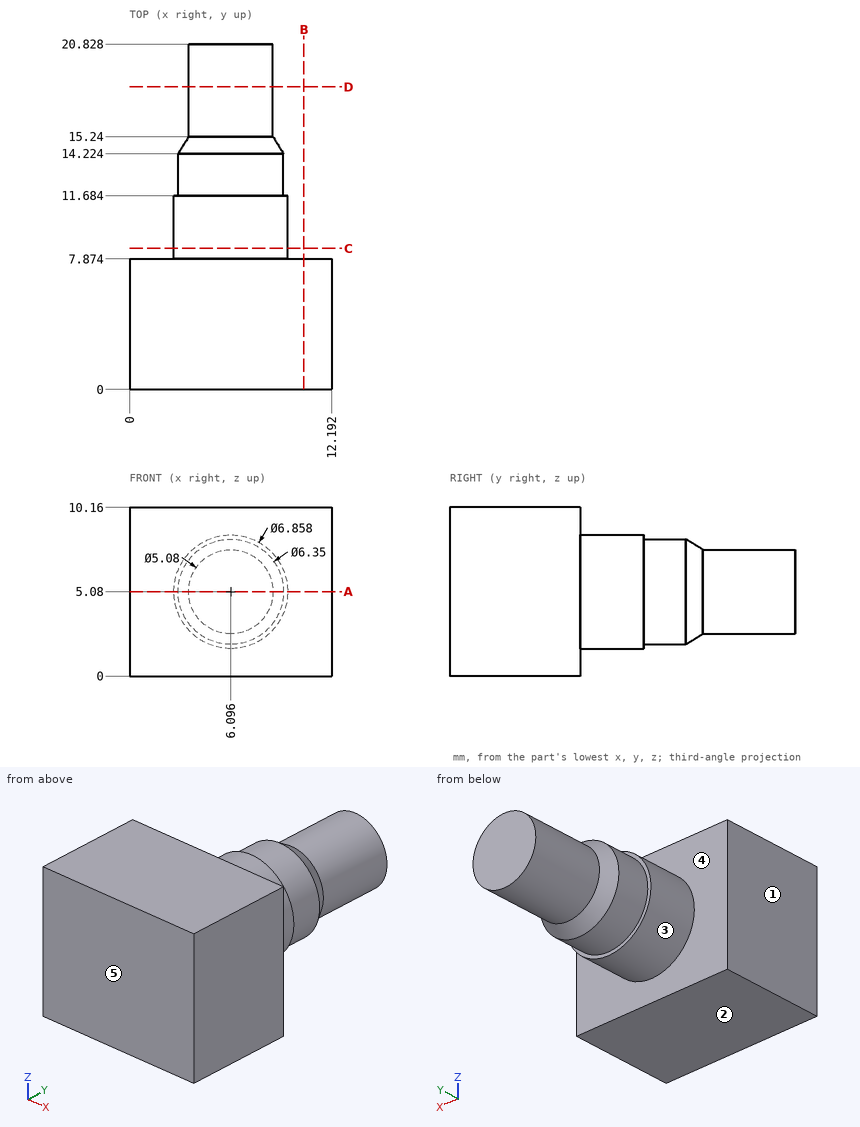
For this review, use the dimensioned drawing (mm, ordinates from the lowest corner) and the shaded views. A direction names the side the tool comes from. Give positions to 0.01 mm unless a question says otherwise; leave off trailing zeros. Order: outer loops, then holes, each group sorted by start corner. A loop starts at its lowest first (then second) coordinate and runs counter-clockwise, first axis right, second up.
1. Mouldability with a two-part tool opening along X and no side actions: class the marked faces 1, 2 and 3 as +X half, -X half, draft (parallel to the pull), parting line (faces both ways), or undercut.
Solution:
face 1: -X half
face 2: draft
face 3: parting line
2. Add section D-D, the plane y = 18.25. State the section outline as (x, z) points, then the cut area to 3 significant figures.
Solution:
outline: circle Ø5.08 at (6.1, 5.08)
area: 20.3 mm2
3. Add section B-B, the plane x = 10.5. State the section outline as (y, z) points.
Solution:
outline: (0, 0) - (7.87, 0) - (7.87, 10.16) - (0, 10.16) - close
4. Tool access review of the marked faces 4 and 5: name each direction out of +Z, -Z, +X, -X, +Y, -Y from which nothing blocks a thin tool from reaching the whole face with its end or side.
Solution:
face 4: +Y
face 5: +Z, -Z, +X, -X, -Y
5. Add section C-C, the plane y = 8.5. State the section outline as (x, z) points.
Solution:
outline: circle Ø6.86 at (6.1, 5.08)
6. For pin 1 Ø6 at (y, z) = (15.5, 6.5) entering from -X; pin 2 Ø5 at (x, y) = (6.5, 14) entering from -Z; pin 3 Ø3 at (y, z) = (9.5, 5) entering from +X (3 decimals), all flat-tipped, find the tip position at first contact; note any pin that passes through.
Solution:
pin 1: stops at x = 2.92
pin 2: stops at z = 1.65
pin 3: stops at x = 9.525
7. Add section A-A, the plane z = 5.08. State the section outline as (x, y) points (3 decimals), then the cut area to 3 significant figures.
Solution:
outline: (0, 0) - (12.192, 0) - (12.192, 7.874) - (9.525, 7.874) - (9.525, 11.684) - (9.271, 11.684) - (9.271, 14.224) - (8.636, 15.24) - (8.636, 20.828) - (3.556, 20.828) - (3.556, 15.24) - (2.921, 14.224) - (2.921, 11.684) - (2.667, 11.684) - (2.667, 7.874) - (0, 7.874) - close
area: 172 mm2
8. To check wall thickness, follow L1, parallel to X at y = 13, z = 5.25; L2, parallel to Y at x = 3.25, z = 9.25; L3, parallel to Z at x = 6.75, y = 15.25. State the ranges of each line that lie inside material, in increasing order.
Solution:
L1: x = 2.93 to 9.27
L2: y = 0 to 7.87
L3: z = 2.63 to 7.53
